Autodesk Inventor part; units mm, degrees
ref_plane "YZ Plane" through (0, 0, 0) normal (1, 0, 0) x (0, 1, 0)
ref_plane "XZ Plane" through (0, 0, 0) normal (0, 1, 0) x (-1, 0, 0)
ref_plane "XY Plane" through (0, 0, 0) normal (0, 0, 1) x (1, 0, 0)
sketch "Sketch1" plane through (0, 0, 0) normal (1, 0, 0) x (0, 1, 0)
  line L0 (5.3982, 6.0675) -> (2.3982, 6.0675)
  line L1 (2.3982, 6.0675) -> (2.3982, -2.9325)
  line L2 (2.3982, -2.9325) -> (5.3982, -2.9325)
  line L3 (5.3982, -2.9325) -> (5.3982, 6.0675)
  point P0 (0, 0)
  dimension "d0" = 3
  dimension "d1" = 9
extrude "Extrusion1" add sketch "Sketch1" along normal mid plane 3
sketch "Sketch2" plane through (-1.5, 2.3982, 6.0675) normal (0, 0, 1) x (1, 0, 0)
  line L0 (0, 3) -> (3, 3)
  line L1 (0, 3) -> (0.5858, 3)
  line L2 (3, 3) -> (3, 0)
  line L3 (3, 0) -> (3, 0.5858)
  line L4 (1.2929, 2.7071) -> (2.7071, 1.2929)
  arc A0 (1.2929, 2.7071) -> (0.5858, 3) centre (0.5858, 2) ccw
  arc A1 (3, 0.5858) -> (2.7071, 1.2929) centre (2, 0.5858) ccw
  line L5 (0.5858, 3) -> (3, 3)
  arc A2 (1.2929, 2.7071) -> (0.5858, 3) centre (0.5858, 2) ccw
  arc A3 (3, 0.5858) -> (2.7071, 1.2929) centre (2, 0.5858) ccw
  line L6 (3, 3) -> (3, 0.5858)
  point P0 (1.5, -2.3982)
  point P1 (1, 3)
  point P2 (3, 1)
  dimension "d5" = 1
extrude "Extrusion2" cut sketch "Sketch2" against normal blind 50
sketch "Sketch4" plane through (-1.5, 0, 0) normal (-1, 0, 0) x (0, 0, 1)
  line L0 (6.0675, 5.3982) -> (-2.9325, 5.3982)
  line L1 (6.0675, 2.3982) -> (-2.9325, 2.3982)
  line L2 (6.0675, 3.6911) -> (-2.9325, 3.6911)
  line L3 (1.5675, 3.6911) -> (2.5531, 5.3982)
  line L4 (1.5675, 3.6911) -> (3.5387, 3.6911) construction
  line L5 (1.5675, 3.6911) -> (0.5819, 5.3982)
  line L6 (0.5819, 5.3982) -> (2.5531, 5.3982)
  point P0 (0, 0)
  dimension "d10" = 60
extrude "Extrusion3" cut sketch "Sketch4" against normal blind 50
sketch "Sketch5" plane through (-1.5, 2.3982, -2.9325) normal (0, -1, 0) x (1, 0, 0)
  line L0 (3, 9) -> (3, 0)
  line L1 (0, 0) -> (0, 9)
  line L2 (0, 6.75) -> (3, 6.75)
  line L3 (0, 2.25) -> (3, 2.25)
  line L4 (0, 2.25) -> (0, 6.75)
  line L5 (3, 2.25) -> (3, 6.75)
  point P0 (1.5, 2.9325)
  point P1 (0, 4.5)
extrude "Extrusion4" add sketch "Sketch5" along normal blind 7
properties part number "parte do segurador de portas"
For this review, take the finished solid that the model builds, in its own axes (mm). A direction names the side the tool comes from. Round coordinates to 2 decimals unless told otherwise and drop trailing zeros. Loops run counter-clockwise (first coordinate to the right, second up) from the corner with the lowest first, then second, coordinate; pieces in that order, holes last.
(1) Clearance check with flat-ended pins moving along their axes: P1, Ø1.1, axis at x = 0.5, z = -2, coming from the -Y side; P2, Ø0.9, axis at x = 0.5, y = -2.5, coming from the -Z side. State where each tip first meets the part, or that it passes through.
Returned:
P1: stops at y = 2.4
P2: stops at z = -0.68
(2) Mouldability with a two-part tool opening along Z and no side actions: class faces 6 (the flat face through (-0.466, 4.343, 1.191)), 7 (the flat face through (0, -1, 3.818)), 8 (the flat face through (0, -1, -0.682)), 9 (the flat face through (-1.5, 1, 2)) as released by +Z, released by -Z, zero draft, split by the parting line, or undercut.
Returned:
face 6: undercut
face 7: released by +Z
face 8: released by -Z
face 9: zero draft
(3) Tool access review of faces 1 (the flat face through (-0.47, 4.34, 1.94)), 2 (the flat face through (1.5, -1, 2)), 3 (the flat face through (0, 2.398, -2)), 4 (the flat face through (0, 2.398, 5)), 5 (the flat face through (0.5, 4.4, 3.8)): name each direction out of +Z, -Z, +X, -X, +Y, -Y from which nothing blocks a thin tool from reaching the whole face with its end or side.
Returned:
face 1: +X, -X, +Y
face 2: +Z, -Z, +X, +Y, -Y
face 3: -Z, +X, -X, -Y
face 4: +Z, +X, -X, -Y
face 5: +Z, -Z, +X, +Y
(4) We need section B-B (z = 5). Give the boundary of the cut face in (x, y).
Returned:
outline: (-1.5, 2.4) - (1.5, 2.4) - (1.5, 2.98) arc R1 ccw to (1.21, 3.69) - (-0.21, 5.11) arc R1 ccw to (-0.91, 5.4) - (-1.5, 5.4) - close
(5) Wall thickness on line 1 along Z through (x, y) = (-0.6, 2.25); line 2 along Y through (x, z) = (-1, 5.75); line 3 along Y through (x, z) = (-0.95, 0.75): over which ranges is each line inside the solid? List them lowest first.
Returned:
line 1: z = -0.68 to 3.82
line 2: y = 2.4 to 5.4
line 3: y = -4.6 to 5.11
(6) We need section D-D (y = 1.25). Give the boundary of the cut face in (x, z).
Returned:
outline: (-1.5, -0.68) - (1.5, -0.68) - (1.5, 3.82) - (-1.5, 3.82) - close
(7) We need section A-A (y = 4.5). Give the boundary of the cut face in (x, z).
Returned:
outline: (-1.5, -2.93) - (0.4, -2.93) - (0.4, 1.1) - (-1.5, 1.1) - close; (-1.5, 2.03) - (0.4, 2.03) - (0.4, 6.07) - (-1.5, 6.07) - close
(8) We need section C-C (x = 0.6). Give the boundary of the cut face in (y, z).
Returned:
outline: (-4.6, -0.68) - (2.4, -0.68) - (2.4, -2.93) - (4.3, -2.93) - (4.3, 1.22) - (3.69, 1.57) - (4.3, 1.92) - (4.3, 6.07) - (2.4, 6.07) - (2.4, 3.82) - (-4.6, 3.82) - close
